```python
from build123d import *

# Parameters (mm, degrees)
F1_DEPTH = 25.4
F2_W     = 36.63072
F2_H     = 17.09543
F3_DEPTH = 50.8
F5_DEPTH = 17.09643
F6_W     = 34.679536
F6_H     = 25.22513
F7_DEPTH = 12.7


with BuildPart() as f1:
    # F0 (on Front) → F1 (new body)
    with BuildSketch(Plane.XZ):
        with BuildLine():
            Line((-9.501953, 38.145531), (-18.31536, 38.145531))
            Line((-18.31536, 38.145531), (-18.31536, -38.145531))
            Line((-18.31536, -38.145531), (18.31536, -38.145531))
            Line((18.31536, -38.145531), (18.31536, 38.145531))
            Line((18.31536, 38.145531), (8.951116, 38.145531))
            Line((8.951116, 38.145531), (8.951116, 15.561176))
            ThreePointArc((8.951116, 15.561176), (-0.275418, 6.334641), (-9.501953, 15.561176))
            Line((-9.501953, 15.561176), (-9.501953, 38.145531))
        make_face()
    extrude(amount=F1_DEPTH)

    # F2 (on face) → F3 (join)
    with BuildSketch(Plane.XZ.offset(25.4)):
        with Locations((0, -29.597816)):
            Rectangle(F2_W, F2_H)
    extrude(amount=F3_DEPTH)

    # F4 (on face) → F5 (cut, through all)
    with BuildSketch(Plane.XY.offset(-21.050101)):
        with BuildLine():
            ThreePointArc((18.31536, -60.358326), (0, -76.070081), (-18.31536, -60.358326))
            Line((-18.31536, -60.358326), (-18.31536, -76.2))
            Line((-18.31536, -76.2), (18.31536, -76.2))
            Line((18.31536, -76.2), (18.31536, -60.358326))
        make_face()
    extrude(amount=-F5_DEPTH, mode=Mode.SUBTRACT)

    # F6 (on face) → F7 (cut)
    with BuildSketch(Plane.YZ.offset(18.31536)):
        with Locations((-17.339768, -25.532966)):
            Rectangle(F6_W, F6_H)
    extrude(amount=-F7_DEPTH, mode=Mode.SUBTRACT)


solid = f1.part
```
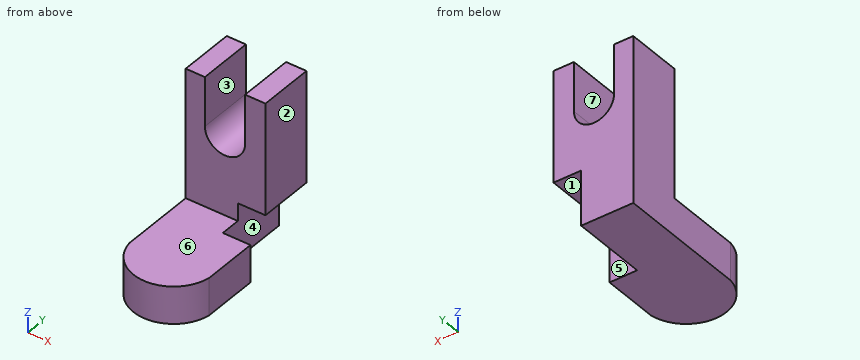
Work out the finished part from the listing and answer in its coordinate system (mm). Face numbers are marked on the shaded views. A direction names the side the tool comes from. Coordinates: 2 decimals unless noted, no trailing zeros. Loops run counter-clockwise (first coordinate to the right, second up) from the corner with the lowest first, then second, coordinate; pieces in that order, holes last. Notation, with made-up numbers: M 54.5,-22.5 L 108.5,-22.5 A19 cw 108.5,4.5 Z; hole C 64.5,42.5 d3. An arc over 180 degrees is marked long. Use CSV: the item, a comma, the result in double quotes. Start each with the question number.
(1) Find section B-B, the plane x = 7. Give the vertices of the cut face in (y, z).
(2) For a pull along X with two mould halves and no side action, classify the marked faces 1, 2 and 3 as +X half, -X half, draft (parallel to the pull), parting line (faces both ways), or undercut.
(3) Find section A-A, the plane z = 21.5. Give the vertices of the cut face in (x, y), then the cut area to 3 significant figures.
(4) Find section D-D, the plane z = 1. Give the vertices of the cut face in (x, y).
(5) Consider line 1 (Z direction, x = -4.5, y = -55.5); line 2 (Y direction, x = -4.5, z = 5.5); line 3 (Z direction, x = 11, y = -11.5). Determine where each line is inside the solid, lowest interval first.
(6) Given pin 1 Ø7.5 at (y, z) = (-10, -25.5) entering from +X; pin 2 Ø12 at (x, z) = (2, -17.5) entering from -Y; pin 3 Ø6.5 at (x, z) = (14.5, -33.5) entering from +Y, each flat-ended and moving along its own axis, determine where each tip first touches the part or whether it passes through.
(7) For the marked faces 4, 5, 6 and 7, determine the directions among +Z, -Z, +X, -X, +Y, -Y from which every point of the face is accessible in a straight line to the end or side of a thin tool.
(8) Find section C-C, the plane y = -19.5. Give the vertices of the cut face in (x, z).
Recorded:
1,outline,"M -74.7,-38.15 L -34.68,-38.15 L -34.68,-21.05 L -74.7,-21.05 Z; M -25.4,-12.92 L 0,-12.92 L 0,9.89 L -25.4,9.89 Z"
2,face 1,"draft"
2,face 2,"+X half"
2,face 3,"undercut"
3,outline,"M -18.32,-25.4 L -9.5,-25.4 L -9.5,0 L -18.32,0 Z; M 8.95,-25.4 L 18.32,-25.4 L 18.32,0 L 8.95,0 Z"
3,area,"462 mm^2"
4,outline,"M -18.32,-25.4 L 18.32,-25.4 L 18.32,0 L -18.32,0 Z"
5,line 1,"z = -38.15 to -21.05"
5,line 2,"y = -25.4 to 0"
5,line 3,"z = -12.92 to 38.15"
6,pin 1,"stops at x = 5.62"
6,pin 2,"stops at y = -76.07"
6,pin 3,"stops at y = -34.68"
7,face 4,"-Z, +X, +Y"
7,face 5,"+Z, -Z, +X, +Y"
7,face 6,"+Z, +X, -X, -Y"
7,face 7,"+Z, +Y, -Y"
8,outline,"M -18.32,-38.15 L 5.62,-38.15 L 5.62,-12.92 L 18.32,-12.92 L 18.32,38.15 L 8.95,38.15 L 8.95,15.56 A9.23 cw -9.5,15.56 L -9.5,38.15 L -18.32,38.15 Z"
